The listing builds one solid part. Answer for the finished solid, in the listing's coordinates (mm). Face numbers are marked on the shaded views. A direction names the side the tool comes from. Coordinates: 2 decimals unless noted, no trailing zeros. Loops run counter-clockwise (first coordinate to the right, second up) from the corner with the lowest first, then second, coordinate; pieces in that order, holes last. Notation, with made-up numbers: M 56.25,83.5 L 105.25,83.5 A21 cw 105.25,113.5 Z; hole C 89,20.25 d5. An arc over 180 degrees is marked long. Answer as a JSON object with one key per item and string values. Group by question number.
1. A cutting plane is placed at C-C on z = 91.5. Give the vertices of the cut face in (x, y).
2. A cutting plane is placed at B-B on z = 30.5. Give the vertices of the cut face in (x, y), and give its area (3 significant figures).
3. For the marked faces 5 and 6, determine the directions among +Z, -Z, +X, -X, +Y, -Y from which every point of the face is accessible in a straight line to the end or side of a thin tool.
4. A cutting plane is placed at D-D on z = 77.5. Give the vertices of the cut face in (x, y).
5. A cutting plane is placed at A-A on x = -25.5. Give the vertices of the cut face in (y, z).
6. Determine the mould class of the marked faces 1, 2, 3 and 4 for opening direction Z: released by +Z, released by -Z, zero draft, split by the parting line, or undercut.
7. Given pin 1 (4 mm diameter, centred on x = -30, y = 15, fed in from -Z); pin 2 (1.5 mm diameter, centred on y = 9.5, z = 124, fed in from +X); pin 3 (14 mm diameter, centred on x = -45.5, z = 36, fed in from +Y); pin 4 (10.5 mm diameter, centred on x = -27, y = 6.5, fed in from +Z), each flat-ended and moving along its own axis, determine where each tip first touches the part or whether it passes through.
8. Straight lines are drawn through the part: L1, parallel to Z at x = -17, y = 13; L2, parallel to Y at x = -48, z = 44; L3, parallel to X at y = 1.5, z = 119. For each, find the intervals that lie inside material, in ascending order.
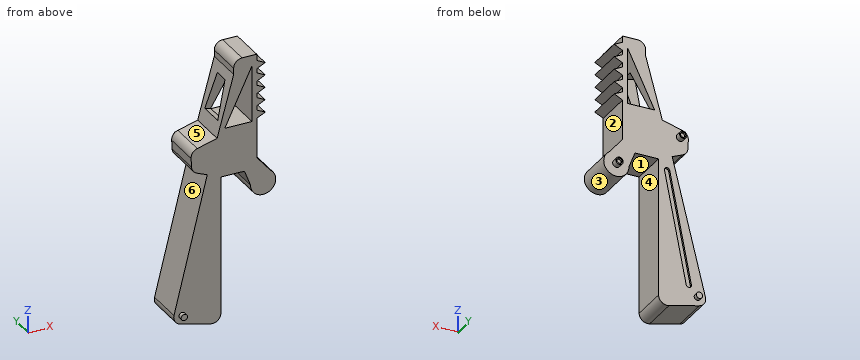
from build123d import *

# Parameters (mm, degrees)
BOSS_EXTRUDE1_DEPTH = 18
FILLET2_R           = 4
BOSS_EXTRUDE2_DEPTH = 18
LPATTERN1_COUNT     = 5
LPATTERN1_PITCH     = 6
CUT_EXTRUDE1_DEPTH  = 26
CUT_EXTRUDE2_DEPTH  = 8
SKETCH6_R           = 1.75
BOSS_EXTRUDE3_DEPTH = 3
SKETCH7_R           = 1.25
CUT_EXTRUDE4_DEPTH  = 1
SKETCH8_R           = 1.25
CUT_EXTRUDE5_DEPTH  = 1
CUT_EXTRUDE6_DEPTH  = 1
SKETCH5_R           = 1.5
BOSS_EXTRUDE4_DEPTH = 2


with BuildPart() as part:
    # Sketch1 → Boss-Extrude1 (new body)
    with BuildSketch(Plane(origin=(0, 0, 0), x_dir=(1, 0, 0), z_dir=(0, 1, 0))):
        Polygon((-40.969304311, -73.71633288), (-34.496108293, -71), (-34.496108293, 0), (-57.792675156, -5.768012861), align=None)
        with BuildLine():
            Line((-23.247974987, -71), (-34.496108293, -71))
            Line((-34.496108293, -71), (-40.969304311, -73.71633288))
            Line((-40.969304311, -73.71633288), (-48.327677264, -76.804110593))
            Line((-48.327677264, -76.804110593), (-48.838396363, -86.791060378))
            Line((-48.838396363, -86.791060378), (-36.286676362, -90.175484262))
            Line((-36.286676362, -90.175484262), (-28.369724317, -119.111998743))
            Line((-28.369724317, -119.111998743), (-28.369724317, -126.111998743))
            Line((-28.369724317, -126.111998743), (-17.369724317, -126.111998743))
            Line((-17.369724317, -126.111998743), (-17.369724317, -76.111998743))
            Line((-17.369724317, -76.111998743), (-10.936329958, -68.456188073))
            ThreePointArc((-10.936329958, -68.456188073), (-11.590696078, -58.200883887), (-20.355503093, -63.56536121))
            Line((-20.355503093, -63.56536121), (-23.247974987, -71))
        make_face()
    extrude(amount=BOSS_EXTRUDE1_DEPTH)

    # Fillet2
    fillet2_edges = [part.edges().sort_by_distance(p)[0] for p in [
        (-57.792675156, 9, 5.768012861),
        (-34.496108293, 9, 0),
        (-28.369724317, 9, 126.111998743),
        (-48.838396363, 9, 86.791060378),
        (-48.327677264, 9, 76.804110593),
    ]]
    fillet(fillet2_edges, radius=FILLET2_R)

    # Sketch2 → Boss-Extrude2 (add, through all)
    with BuildSketch(Plane(origin=(0, 18, 0), x_dir=(1, 0, 0), z_dir=(0, 1, 0))):
        Polygon((-17.369724317, -119.111998743), (-17.369724317, -123.111998743), (-13.369724317, -121.111998743), align=None)
    boss_extrude2 = extrude(amount=-BOSS_EXTRUDE2_DEPTH)

    # LPattern1: Boss-Extrude2 ×5
    with Locations(*[(0, 0, -i * LPATTERN1_PITCH) for i in range(1, LPATTERN1_COUNT)]):
        add(boss_extrude2)

    # Sketch3 → Cut-Extrude1 (cut)
    with BuildSketch(Plane(origin=(0, 18, 0), x_dir=(1, 0, 0), z_dir=(0, 1, 0))):
        Polygon((-19.631839037, -121.116880753), (-19.631839037, -94.116880753), (-32.631839037, -94.116880753), align=None)
    extrude(amount=-CUT_EXTRUDE1_DEPTH, mode=Mode.SUBTRACT)

    # Sketch4 → Cut-Extrude2 (cut)
    with BuildSketch(Plane(origin=(-56.713154452, 0, 15.516565563), x_dir=(0.2638984014912162, 0, 0.9645504827070385), z_dir=(-0.9645504827070386, 0, 0.2638984014912162))):
        Polygon((84.402810986, 15), (84.402810986, 3), (102.402810986, 5.456363489), (102.402810986, 12.543636511), align=None)
    extrude(amount=-CUT_EXTRUDE2_DEPTH, mode=Mode.SUBTRACT)

    # Sketch6 → Boss-Extrude3 (add)
    with BuildSketch(Plane(origin=(0, 18, 0), x_dir=(1, 0, 0), z_dir=(0, 1, 0))):
        with Locations(Location((-14.355633277, -63.525836684, 0), (0, 0, 270))):
            Circle(SKETCH6_R)
        with Locations(Location((-44.67866751, -83.769823901, 0), (0, 0, 270))):
            Circle(SKETCH6_R)
    extrude(amount=BOSS_EXTRUDE3_DEPTH)

    # Sketch7 → Cut-Extrude4 (cut)
    with BuildSketch(Plane(origin=(0, 21, 0), x_dir=(1, 0, 0), z_dir=(0, 1, 0))):
        with Locations(Location((-14.355633277, -63.525836684, 0), (0, 0, 270))):
            Circle(SKETCH7_R)
    extrude(amount=-CUT_EXTRUDE4_DEPTH, mode=Mode.SUBTRACT)

    # Sketch8 → Cut-Extrude5 (cut)
    with BuildSketch(Plane(origin=(0, 21, 0), x_dir=(1, 0, 0), z_dir=(0, 1, 0))):
        with Locations(Location((-44.67866751, -83.769823901, 0), (0, 0, 270))):
            Circle(SKETCH8_R)
    extrude(amount=-CUT_EXTRUDE5_DEPTH, mode=Mode.SUBTRACT)

    # Sketch9 → Cut-Extrude6 (cut)
    with BuildSketch(Plane(origin=(0, 18, 0), x_dir=(1, 0, 0), z_dir=(0, 1, 0))):
        with BuildLine():
            Line((-47.653198818, -13.430984589), (-37.315061162, -66.229330476))
            ThreePointArc((-37.315061162, -66.229330476), (-38.31592464, -67.717570951), (-39.804165115, -66.716707473))
            Line((-39.804165115, -66.716707473), (-50.142302771, -13.918361587))
            ThreePointArc((-50.142302771, -13.918361587), (-49.141439293, -12.430121111), (-47.653198818, -13.430984589))
        make_face()
    extrude(amount=-CUT_EXTRUDE6_DEPTH, mode=Mode.SUBTRACT)

    # Sketch5 → Boss-Extrude4 (add)
    with BuildSketch(Plane(origin=(0, 18, 0), x_dir=(1, 0, 0), z_dir=(0, 1, 0))):
        with Locations(Location((-52.948578536, -8.689438528, 0), (0, 0, 270))):
            Circle(SKETCH5_R)
    boss_extrude4 = extrude(amount=BOSS_EXTRUDE4_DEPTH)

    # Mirror1: Boss-Extrude4 across plane
    add(boss_extrude4.mirror(Plane.ZX.offset(9)))


solid = part.part
From the geometry:
{
 "1": {"outline": "M -35.92,0 L -17.37,0 L -17.37,18 L -35.92,18 Z"},
 "2": {"outline": "M -51.67,0 L -34.5,0 L -34.5,18 L -44.31,18 L -44.31,17 L -46.9,17 L -46.9,18 L -51.67,18 Z", "area": "307 mm²"},
 "3": {"face 5": "+Z, -X, +Y, -Y", "face 6": "-X, +Y, -Y"},
 "4": {"outline": "M -47.91,0 L -17.37,0 L -17.37,18 L -47.91,18 Z"},
 "5": {"outline": "M 0,71 L 18,71 L 18,94.12 L 0,94.12 Z; M 0,108.93 L 4.9,108.93 L 5.46,113.14 L 12.54,113.14 L 13.1,108.93 L 18,108.93 L 18,125.95 L 0,125.95 Z"},
 "6": {"face 1": "released by -Z", "face 2": "undercut", "face 3": "split by the parting line", "face 4": "zero draft"},
 "7": {"pin 1": "stops at z = 71", "pin 2": "stops at x = -17.37", "pin 3": "stops at y = 18", "pin 4": "stops at z = 126.11"},
 "8": {"L1": "z = 58.14 to 75.67, 95.3 to 98.93, 101.3 to 104.93, 107.3 to 110.93, 113.3 to 116.93, 119.3 to 122.93", "L2": "y = 0 to 18", "L3": "x = -28.4 to -20.65, -19.63 to -17.37"}
}
